from build123d import *

# Parameters (mm, degrees)
F2_SIZE  = 5.08
F3_R     = 6.35
F4_DEPTH = 127
F5_DEPTH = 177.8


with BuildPart() as f1:
    # F0 (on Front) → F1 (revolve)
    with BuildSketch(Plane.XZ):
        with BuildLine():
            Line((-38.1, 0), (0, 0))
            Line((0, 0), (0, 19.05))
            ThreePointArc((0, 19.05), (-6.35, 25.4), (0, 31.75))
            Line((0, 31.75), (0, 69.85))
            ThreePointArc((0, 69.85), (-6.35, 76.2), (0, 82.55))
            Line((0, 82.55), (0, 101.6))
            Line((0, 101.6), (-38.1, 101.6))
            Line((-38.1, 101.6), (-38.1, 0))
        make_face()
    revolve(axis=Axis((-38.1, 0, 50.8), (0, 0, 1)))

    # F2
    f2_edges = [f1.edges().sort_by_distance(p)[0] for p in [
        (-76.2, 0, 101.6),
        (-76.2, 0, 0),
    ]]
    chamfer(f2_edges, length=F2_SIZE)

    # F3 (on Front) → F4 (cut)
    with BuildSketch(Plane.XZ):
        with Locations((-38.1, 50.8)):
            Circle(F3_R)
    extrude(amount=-F4_DEPTH, mode=Mode.SUBTRACT)

    # F5 (add): a face of the model
    f5_faces = [f1.faces().sort_by_distance(p)[0] for p in [
        (-38.1, 0, 50.8),
    ]]
    extrude(f5_faces, amount=F5_DEPTH)


solid = f1.part
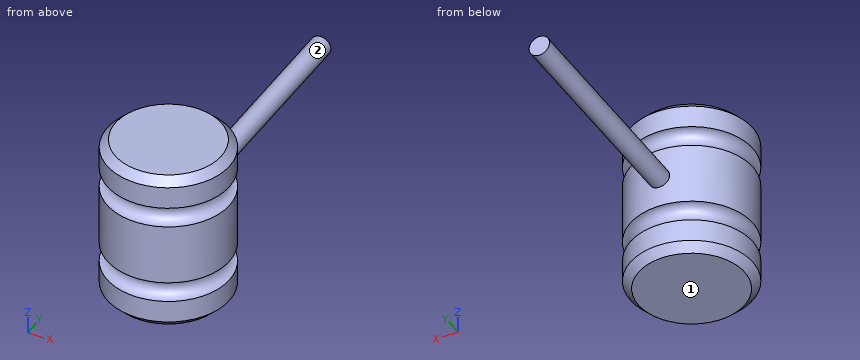
The listing builds one solid part. Answer for the finished solid, in the listing's coordinates (mm). Face numbers are marked on the shaded views. A direction names the side the tool comes from. Give positions to 0.01 mm unless a question says otherwise; leave off trailing zeros. Write each loop counter-clockwise with the first axis right and the second up, starting at its lowest first coordinate (ties: lowest second). Pieces come first, ordered by that corner, then holes.
1) Section D-D (y = 149) is taken. Write down the section's boundary in (x, z).
2) Given P1, Ø6, axis at x = -49, z = 69, coming from the +Y side; P2, Ø10, axis at x = -46.5, z = 63, coming from the +Y side; P3, Ø1, axis at x = -35.5, z = 28, coming from the -Y side, each flat-ended and moving along its own axis, determine where each tip first touches the part or whether it passes through.
3) Section A-A (y = 0) is taken. Write down the section's boundary in (x, z), and give its area (3 significant figures).
4) Section C-C (z = 50.8) is taken. Write down the section's boundary in (x, y), and give its area (3 significant figures).
5) Section B-B (x = -38.1) is taken. Write down the section's boundary in (y, z), and give its area (3 significant figures).
6) Find the intervals of material crossed by L1, parallel to Z at x = -68.5, y = 16; L2, parallel to Z at x = -70, y = 10; L3, parallel to Y at x = -3.5, z = 35.5, in increasing order.
7) A tool of negligible diameter and unlimited length cuts with its end or side. For the marked faces 1 and 2, from which of +Z, -Z, +X, -X, +Y, -Y can it reach the whole face along a straight path? Write none if from no direction.
Response:
1. outline: circle Ø12.7 at (-38.1, 50.8)
2. P1: stops at y = 37.27
2. P2: stops at y = 37.95
2. P3: stops at y = -32.46
3. outline: (-76.2, 5.08) - (-71.12, 0) - (-5.08, 0) - (0, 5.08) - (0, 19.05) arc R6.35 cw to (0, 31.75) - (0, 69.85) arc R6.35 cw to (0, 82.55) - (0, 96.52) - (-5.08, 101.6) - (-71.12, 101.6) - (-76.2, 96.52) - (-76.2, 82.55) arc R6.35 cw to (-76.2, 69.85) - (-76.2, 31.75) arc R6.35 cw to (-76.2, 19.05) - close
3. area: 7,440 mm2
4. outline: (-44.45, 37.57) arc R38.1 ccw (long way) to (-31.75, 37.57) - (-31.75, 177.8) - (-44.45, 177.8) - close
4. area: 6,340 mm2
5. outline: (-38.1, 5.08) - (-33.02, 0) - (33.02, 0) - (38.1, 5.08) - (38.1, 19.05) arc R6.35 cw to (38.1, 31.75) - (38.1, 44.45) - (177.8, 44.45) - (177.8, 57.15) - (38.1, 57.15) - (38.1, 69.85) arc R6.35 cw to (38.1, 82.55) - (38.1, 96.52) - (33.02, 101.6) - (-33.02, 101.6) - (-38.1, 96.52) - (-38.1, 82.55) arc R6.35 cw to (-38.1, 69.85) - (-38.1, 31.75) arc R6.35 cw to (-38.1, 19.05) - close
5. area: 9,210 mm2
6. L1: z = 1.33 to 20.27, 30.53 to 71.07, 81.33 to 100.27
6. L2: z = 0.41 to 21.1, 29.7 to 71.9, 80.5 to 101.19
6. L3: y = -15.95 to 15.95
7. face 1: -Z, +X, -X, +Y, -Y
7. face 2: +Y
